```python
from build123d import *

# Parameters (mm, degrees)
SKETCH1_W                = 205.74
SKETCH1_H                = 205.74
SKETCH1_R                = 2.200000045
BOSS_EXTRUDE1_DEPTH      = 6.35
SKETCH3_R                = 9.999999939
CUT_EXTRUDE2_DEPTH       = 146.618667416
SKETCH4_W                = 69.85
SKETCH4_H                = 69.85
CUT_EXTRUDE3_DEPTH       = 146.618667416
FILLET4_R                = 6.35
CIRPATTERN6_COUNT        = 4
FILLET4_OF_CIRPATTERN6_R = 6.35
FILLET8_R                = 38.1
FILLET9_R                = 76.2
SKETCH10_R               = 2.099999991
CUT_EXTRUDE6_DEPTH       = 146.618667416
SKETCH11_R               = 4.000000001
CUT_EXTRUDE7_DEPTH       = 3.000000096
CIRPATTERN4_COUNT        = 4


with BuildPart() as part:
    # Sketch1 → Boss-Extrude1 (new body)
    with BuildSketch(Plane(origin=(0, 0, 0), x_dir=(1, 0, 0), z_dir=(0, 1, 0))):
        Rectangle(SKETCH1_W, SKETCH1_H)
        with Locations(Location((63.5, 0, 0), (0, 0, 270))):
            Circle(SKETCH1_R, mode=Mode.SUBTRACT)
        with Locations(Location((0, -63.5, 0), (0, 0, 270))):
            Circle(SKETCH1_R, mode=Mode.SUBTRACT)
        with Locations(Location((-63.5, 0, 0), (0, 0, 270))):
            Circle(SKETCH1_R, mode=Mode.SUBTRACT)
        with Locations(Location((0, 63.5, 0), (0, 0, 270))):
            Circle(SKETCH1_R, mode=Mode.SUBTRACT)
    extrude(amount=BOSS_EXTRUDE1_DEPTH)

    # Sketch3 → Cut-Extrude2 (cut, through all)
    with BuildSketch(Plane(origin=(0, 6.35, 0), x_dir=(1, 0, 0), z_dir=(0, 1, 0))):
        with Locations(Location((0, 0, 0), (0, 0, 270))):
            Circle(SKETCH3_R)
    extrude(amount=-CUT_EXTRUDE2_DEPTH, mode=Mode.SUBTRACT)

    # Sketch4 → Cut-Extrude3 (cut, through all)
    with BuildSketch(Plane(origin=(0, 6.35, 0), x_dir=(1, 0, 0), z_dir=(0, 1, 0))):
        with Locations((-44.901280605, 44.901280605)):
            Rectangle(SKETCH4_W, SKETCH4_H)
    cut_extrude3 = extrude(amount=-CUT_EXTRUDE3_DEPTH, mode=Mode.SUBTRACT)

    # Fillet4
    fillet4_edges = [part.edges().sort_by_distance(p)[0] for p in [
        (-9.976280605, 3.175, -79.826280605),
        (-9.976280605, 3.175, -9.976280605),
        (-79.826280605, 3.175, -9.976280605),
    ]]
    fillet(fillet4_edges, radius=FILLET4_R)

    # CirPattern6: Cut-Extrude3 ×4 about axis
    cirpattern6_axis = Axis((0, 0, 0), (0, 1, 0))
    for i in range(1, CIRPATTERN6_COUNT):
        add(cut_extrude3.rotate(cirpattern6_axis, i * 360 / CIRPATTERN6_COUNT), mode=Mode.SUBTRACT)

    # Fillet4 of CirPattern6
    fillet4_of_cirpattern6_edges = [part.edges().sort_by_distance(p)[0] for p in [
        (-79.826280605, 3.175, 9.976280605),
        (-9.976280605, 3.175, 9.976280605),
        (-9.976280605, 3.175, 79.826280605),
        (9.976280605, 3.175, 79.826280605),
        (9.976280605, 3.175, 9.976280605),
        (79.826280605, 3.175, 9.976280605),
        (79.826280605, 3.175, -9.976280605),
        (9.976280605, 3.175, -9.976280605),
        (9.976280605, 3.175, -79.826280605),
    ]]
    fillet(fillet4_of_cirpattern6_edges, radius=FILLET4_OF_CIRPATTERN6_R)

    # Fillet8
    fillet8_edges = [part.edges().sort_by_distance(p)[0] for p in [
        (-79.826280605, 3.175, -79.826280605),
        (79.826280605, 3.175, -79.826280605),
        (79.826280605, 3.175, 79.826280605),
        (-79.826280605, 3.175, 79.826280605),
    ]]
    fillet(fillet8_edges, radius=FILLET8_R)

    # Fillet9
    fillet9_edges = [part.edges().sort_by_distance(p)[0] for p in [
        (102.87, 3.175, 102.87),
        (-102.87, 3.175, 102.87),
        (-102.87, 3.175, -102.87),
        (102.87, 3.175, -102.87),
    ]]
    fillet(fillet9_edges, radius=FILLET9_R)

    # Sketch10 → Cut-Extrude6 (cut, through all)
    with BuildSketch(Plane(origin=(0, 6.35, 0), x_dir=(1, 0, 0), z_dir=(0, 1, 0))):
        with Locations(Location((0, -26.035, 0), (0, 0, 270))):
            Circle(SKETCH10_R)
        with Locations(Location((0, -76.835, 0), (0, 0, 270))):
            Circle(SKETCH10_R)
        with Locations(Location((-19.05, -97.79, 0), (0, 0, 270))):
            Circle(SKETCH10_R)
        with Locations(Location((19.05, -97.79, 0), (0, 0, 270))):
            Circle(SKETCH10_R)
    cut_extrude6 = extrude(amount=-CUT_EXTRUDE6_DEPTH, mode=Mode.SUBTRACT)

    # Sketch11 → Cut-Extrude7 (cut)
    with BuildSketch(Plane.XZ):
        with Locations(Location((-19.05, 97.79, 0), (0, 0, 270))):
            Circle(SKETCH11_R)
        with Locations(Location((19.05, 97.79, 0), (0, 0, 270))):
            Circle(SKETCH11_R)
        with Locations(Location((0, 76.835, 0), (0, 0, 270))):
            Circle(SKETCH11_R)
        with Locations(Location((0, 26.035, 0), (0, 0, 270))):
            Circle(SKETCH11_R)
    cut_extrude7 = extrude(amount=-CUT_EXTRUDE7_DEPTH, mode=Mode.SUBTRACT)

    # CirPattern4: Cut-Extrude6, Cut-Extrude7 ×4 about axis
    cirpattern4_axis = Axis((0, 0, 0), (0, 1, 0))
    add([cut_extrude6.rotate(cirpattern4_axis, i * 360 / CIRPATTERN4_COUNT) for i in range(1, CIRPATTERN4_COUNT)], mode=Mode.SUBTRACT)
    add([cut_extrude7.rotate(cirpattern4_axis, i * 360 / CIRPATTERN4_COUNT) for i in range(1, CIRPATTERN4_COUNT)], mode=Mode.SUBTRACT)


solid = part.part
```
Check sheet for the modelled part. Datum: model origin and axes. Units: mm. A direction names the side the tool comes from. Round coordinates to 2 decimals unless told otherwise and drop trailing zeros. Write each loop counter-clockwise with the first axis right and the second up, starting at its lowest first coordinate (ties: lowest second). Pieces come first, ordered by that corner, then holes. Notation, with made-up numbers: (70, -4) -> (120, -4) arc R23 ccw to (120, 27) -> close; hole circle Ø7 at (30, 3.5). An arc over 180 degrees is marked (long way). Put each result on its own line as item: value.
(1) Mould release check, pull along X, two halves, no side actions. Record for faces 3 (the face through (-81.1, 3.2, -80)), 4 (the face through (0.18, 1.48, 80.83)), 5 (the face through (0, 3, 102.87)): released by +X, released by -X, zero draft, split by the parting line, or undercut.
Values found:
face 3: released by -X
face 4: undercut
face 5: zero draft
(2) Go/stop test with flat-tipped pins: pin 1 Ø6.5 at (x, z) = (97.79, 19.05) entering from -Y; pin 2 Ø2 at (y, z) = (2, 66) entering from +X; pin 3 Ø4 at (x, z) = (-97.79, -19.05) entering from -Y; pin 4 Ø3 at (y, z) = (3.5, -51) entering from -X. Record where each tip stops, or that it passes through.
Values found:
pin 1: stops at y = 3
pin 2: stops at x = 92.53
pin 3: passes through
pin 4: stops at x = -99.37
(3) Sectioned sample at A-A (x = 38). Enter the section's corners in (y, z), plus the area to 3 significant figures.
Values found:
outline: (0, -102.02) -> (6.35, -102.02) -> (6.35, -79.83) -> (0, -79.83) -> close; (0, -9.98) -> (6.35, -9.98) -> (6.35, 9.98) -> (0, 9.98) -> close; (0, 79.83) -> (6.35, 79.83) -> (6.35, 102.02) -> (0, 102.02) -> close
area: 409 mm^2
(4) Material ranges on line 1 (Z direction, x = 28.5, y = 3.25); line 2 (X direction, y = 5, z = -76); line 3 (Z direction, x = 29.5, y = 2.25), recorded low to high.
Values found:
line 1: z = -102.85 to -79.83, -9.98 to 9.98, 79.83 to 102.85
line 2: x = -84.75 to -58.37, -10.5 to -1.93, 1.93 to 10.5, 58.37 to 84.75
line 3: z = -102.82 to -79.83, -9.98 to -2, 2 to 9.98, 79.83 to 102.82
(5) Tool access check on faces 1 (the face through (68.96, 3.13, 68.37)), 2 (the face through (24, 3, 2)). Record the directions out of +Z, -Z, +X, -X, +Y, -Y that give a thin tool (end or side, any length) a straight path to the whole face; none if there is none.
Values found:
face 1: +Y, -Y
face 2: -Y
(6) Sectioned sample at B-B (y = 2). Count the separate pieces of the cut face and the enclosed holes in it, plus the area to 3 significant figures.
Values found:
separate pieces: 1
enclosed holes: 25
area: 18,000 mm^2
(7) Sectioned sample at C-C (z = 84). Enter the section's corners in (x, y), plus the area to 3 significant figures.
Values found:
outline: (-76.87, 0) -> (76.87, 0) -> (76.87, 6.35) -> (-76.87, 6.35) -> close
area: 976 mm^2
